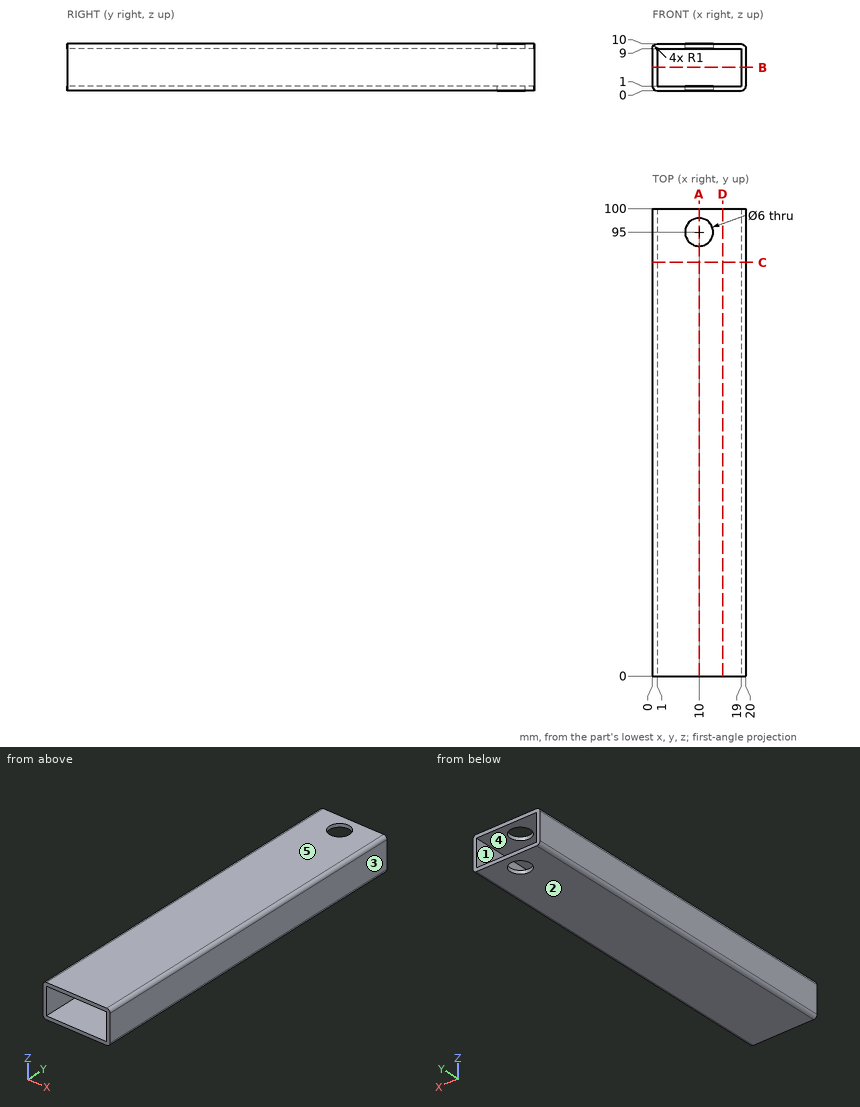
Input: dimensioned drawing with shaded views. Units: mm. Origin: part minimum x, y, z. A direction names the side the tool comes from. Coordinates: 2 decimals unless noted, no trailing zeros. Loops run counter-clockwise (first coordinate to the right, second up) from the corner with the lowest first, then second, coordinate; pieces in that order, holes last. Notation, with made-up numbers: M 36.25,82 L 58.25,82 A16 cw 58.25,92 Z; hole C 43,-21 d11. An arc over 180 degrees is marked long. One line per item, written item: value. Start each with the question number.
1) Cut plane C-C (y = 88.5). Return loops of the section in (x, z).
2) Cut plane D-D (x = 15). Return loops of the section in (y, z).
3) Pin query (flat end, axial travel): P1, Ø8, axis at x = 10, y = 95, coming from the +Z side. Return the tip coordinate at first contact, or that it passes through.
4) Cut plane A-A (x = 10). Return loops of the section in (y, z).
5) Cut plane B-B (z = 5). Return loops of the section in (x, y).
6) Reachability of the marked faces 1 and 2 from +Z, -Z, +X, -X, +Y, -Y: full face, straight path, thin tool, end or side. Return the list, or none.
7) Draft query along X for the marked faces 3, 4 and 5. Return one class per face: released by +X, released by -X, zero draft, split by the parting line, or undercut.
8) Material intervals for L1, parallel to Z at x = 6, y = 72; L2, parallel to Y at x = 10, z = 9.5; L3, parallel to X at y = 71.5, z = 3.25, sorted ascending. Write a range as from..to.
Evaluation:
1. outline: M 0,1 A1 ccw 1,0 L 19,0 A1 ccw 20,1 L 20,9 A1 ccw 19,10 L 1,10 A1 ccw 0,9 Z; hole M 1,1 L 19,1 L 19,9 L 1,9 Z
2. outline: M 0,0 L 100,0 L 100,1 L 0,1 Z; M 0,9 L 100,9 L 100,10 L 0,10 Z
3. P1: z = 10
4. outline: M 0,0 L 92,0 L 92,1 L 0,1 Z; M 0,9 L 92,9 L 92,10 L 0,10 Z; M 98,0 L 100,0 L 100,1 L 98,1 Z; M 98,9 L 100,9 L 100,10 L 98,10 Z
5. outline: M 0,0 L 1,0 L 1,100 L 0,100 Z; M 19,0 L 20,0 L 20,100 L 19,100 Z
6. face 1: +Y, -Y
6. face 2: -Z, +X, -X, +Y, -Y
7. face 3: released by +X
7. face 4: undercut
7. face 5: zero draft
8. L1: 0..1, 9..10
8. L2: 0..92, 98..100
8. L3: 0..1, 19..20
